from build123d import *

# Parameters (mm, degrees)
SKETCH1_W                       = 16
SKETCH1_H                       = 3.2
BOSS_EXTRUDE1_DEPTH             = 15.8
SKETCH2_R                       = 2.4
BOSS_EXTRUDE2_DEPTH             = 1.6
LPATTERN1_COUNT                 = 2
LPATTERN1_PITCH                 = 8
LPATTERN1_COUNT_DIR2            = 6
LPATTERN1_PITCH_DIR2            = 8
SHELL1_T                        = -1.2
SKETCH3_R                       = 3.25
SKETCH3_R_2                     = 2.4
BOSS_EXTRUDE3_DEPTH             = 1.8
SHELL2_START                    = -14.6
SHELL2_DEPTH                    = 13.4
BOSS_EXTRUDE4_REACH             = 32.137
SKETCH11_R                      = 2.4
SKETCH11_R_2                    = 1.55
BOSS_EXTRUDE4_DIRECTION_2_DEPTH = 1.6
SHELL6_T                        = -1.2


# Read off the part's stored shape, not the designer's step: Shell2
with BuildPart() as part:
    # Sketch1 → Boss-Extrude1 (new body)
    with BuildSketch(Plane.XY):
        with Locations((8, 1.6)):
            Rectangle(SKETCH1_W, SKETCH1_H)
    extrude(amount=-BOSS_EXTRUDE1_DEPTH)

    # Sketch2 → Boss-Extrude2 (add)
    with BuildSketch(Plane(origin=(0, 3.2, 0), x_dir=(1, 0, 0), z_dir=(0, 1, 0))):
        with Locations(Location((3.9, 3.9, 0), (0, 0, 270))):
            Circle(SKETCH2_R)
    boss_extrude2 = extrude(amount=BOSS_EXTRUDE2_DEPTH)

    # LPattern1: Boss-Extrude2 2 × 6, 8 skipped
    with Locations(*[(j * LPATTERN1_PITCH_DIR2, 0, -i * LPATTERN1_PITCH) for i in range(LPATTERN1_COUNT) for j in range(LPATTERN1_COUNT_DIR2) if (i, j) not in ((0, 0), (0, 2), (0, 3), (0, 4), (0, 5), (1, 2), (1, 3), (1, 4), (1, 5))]):
        add(boss_extrude2)

    # Shell1
    shell1_openings = [part.faces().sort_by_distance(p)[0] for p in [
        (8, 0, -7.9),
    ]]
    offset(amount=SHELL1_T, openings=shell1_openings, kind=Kind.INTERSECTION)

    # Sketch3 → Boss-Extrude3 (add)
    with BuildSketch(Plane.XZ.offset(-2)):
        with Locations(Location((7.9, -7.9, 0), (0, 0, 90))):
            Circle(SKETCH3_R)
        with Locations(Location((7.9, -7.9, 0), (0, 0, 270))):
            Circle(SKETCH3_R_2, mode=Mode.SUBTRACT)
    extrude(amount=BOSS_EXTRUDE3_DEPTH)

    # Sketch7 → Loft1 section 0
    with BuildSketch(Plane(origin=(23.8, 0, 0), x_dir=(0, 0, -1), z_dir=(1, 0, 0))):
        with BuildLine():
            Line((15.8, 9.6), (15.8, 8.4))
            Line((15.8, 8.4), (0, 8.4))
            Line((0, 8.4), (0, 9.6))
            Line((0, 9.6), (15.8, 9.6))
        make_face()
    # Sketch5 → Loft1 section 1
    with BuildSketch(Plane(origin=(16, 0, 0), x_dir=(0, 0, -1), z_dir=(1, 0, 0))):
        with BuildLine():
            Line((0, 0), (0, 9.6))
            Line((0, 9.6), (15.8, 9.6))
            Line((15.8, 9.6), (15.8, 0))
            Line((15.8, 0), (0, 0))
        make_face()
    loft1 = loft()

    # Shell2 outline → Shell2 (cut)
    with BuildSketch(Plane.XY.offset(SHELL2_START)):
        Polygon((16, 1.763535985), (16.219573728, 2), (16, 2), align=None)
        Polygon((17.2, 9.6), (17.2, 3.055843678), (22.6, 8.871228293), (22.6, 9.6), align=None)
    extrude(amount=SHELL2_DEPTH, mode=Mode.SUBTRACT)

    # Sketch11 → Boss-Extrude4 (add, up to next)
    with BuildSketch(Plane(origin=(0, 9.6, 0), x_dir=(1, 0, 0), z_dir=(0, 1, 0)), mode=Mode.PRIVATE) as boss_extrude4_sk1:
        with Locations(Location((19.9, 11.9, 0), (0, 0, 180))):
            Circle(SKETCH11_R)
        with Locations((19.9, 11.9)):
            Circle(SKETCH11_R_2, mode=Mode.SUBTRACT)
    boss_extrude4_tool1 = extrude(boss_extrude4_sk1.sketch, amount=-BOSS_EXTRUDE4_REACH, mode=Mode.PRIVATE) - part.part
    # Sketch11 → Boss-Extrude4 (add, up to next)
    with BuildSketch(Plane(origin=(0, 9.6, 0), x_dir=(1, 0, 0), z_dir=(0, 1, 0)), mode=Mode.PRIVATE) as boss_extrude4_sk2:
        with Locations(Location((19.9, 3.9, 0), (0, 0, 180))):
            Circle(SKETCH11_R)
        with Locations((19.9, 3.9)):
            Circle(SKETCH11_R_2, mode=Mode.SUBTRACT)
    boss_extrude4_tool2 = extrude(boss_extrude4_sk2.sketch, amount=-BOSS_EXTRUDE4_REACH, mode=Mode.PRIVATE) - part.part
    boss_extrude4_1 = boss_extrude4_tool1.solids().sort_by_distance((22.232118, 9.6, -11.9))[0]
    add(boss_extrude4_1)
    boss_extrude4_2 = boss_extrude4_tool2.solids().sort_by_distance((22.232118, 9.6, -3.9))[0]
    add(boss_extrude4_2)
    boss_extrude4 = boss_extrude4_1 + boss_extrude4_2  # Boss-Extrude4 as one shape, for the pattern or mirror that repeats it

    # Sketch11 → Boss-Extrude4 direction 2 (add)
    # profile 1 of 2: a face of its own
    with BuildSketch(Plane(origin=(0, 9.6, 0), x_dir=(1, 0, 0), z_dir=(0, 1, 0))):
        with Locations(Location((19.9, 11.9, 0), (0, 0, 180))):
            Circle(SKETCH11_R)
        with Locations((19.9, 11.9)):
            Circle(SKETCH11_R_2, mode=Mode.SUBTRACT)
    # profile 2 of 2: a face of its own
    with BuildSketch(Plane(origin=(0, 9.6, 0), x_dir=(1, 0, 0), z_dir=(0, 1, 0))):
        with Locations(Location((19.9, 3.9, 0), (0, 0, 180))):
            Circle(SKETCH11_R)
        with Locations((19.9, 3.9)):
            Circle(SKETCH11_R_2, mode=Mode.SUBTRACT)
    boss_extrude4_direction_2 = extrude(amount=BOSS_EXTRUDE4_DIRECTION_2_DEPTH)

    # Mirror1: Loft1 across plane
    add(loft1.mirror(Plane(origin=(8, 0, 0), x_dir=(0, 0, 1), z_dir=(1, 0, 0))))


with BuildPart() as body_2:
    # Split1: the piece on the far side of the plane
    add(part.part)
    split(bisect_by=Plane(origin=(0, 0, 0), x_dir=(0, 0, 1), z_dir=(1, 0, 0)), keep=Keep.BOTTOM)

    # Shell6
    shell6_openings = [body_2.faces().sort_by_distance(p)[0] for p in [
        (-3.9, 9.6, -7.9),
    ]]
    offset(amount=SHELL6_T, openings=shell6_openings, kind=Kind.INTERSECTION)


with BuildPart() as part_1:
    add(part.part)

    # Split1
    split(bisect_by=Plane(origin=(0, 0, 0), x_dir=(0, 0, 1), z_dir=(1, 0, 0)), keep=Keep.TOP)


with BuildPart() as body_2_1:
    add(body_2.part)

    # Combine1: union part
    add(part_1.part)

    # Mirror4: Boss-Extrude4, Boss-Extrude4 direction 2 across plane
    add(boss_extrude4.mirror(Plane(origin=(8, 0, 0), x_dir=(0, 0, 1), z_dir=(1, 0, 0))))
    add(boss_extrude4_direction_2.mirror(Plane(origin=(8, 0, 0), x_dir=(0, 0, 1), z_dir=(1, 0, 0))))


solid = body_2_1.part
Verification items for the finished model (mm, model axes). A direction names the side the tool comes from. Give positions to 0.01 mm unless a question says otherwise; leave off trailing zeros. Write each loop counter-clockwise with the first axis right and the second up, starting at its lowest first coordinate (ties: lowest second). Pieces come first, ordered by that corner, then holes. Notation, with made-up numbers: (66, -1) - (119, -1) arc R19 ccw to (119, 25) - close; hole circle Ø5 at (-16.5, -10.75). An arc over 180 degrees is marked (long way). Answer as CSV lines item,"result". Start each with the question number.
1. Depth check by flat-ended pin: pin 1 (1.9 mm diameter, centred on x = 3.9, z = -11.9, fed in from +Y); pin 2 (2 mm diameter, centred on x = 4, y = 4.5, fed in from -Z); pin 3 (1.5 mm diameter, centred on x = -4, z = -7, fed in from -Y). Enter the tip coordinate at first touch or a pass-through.
2. Sectioned sample at B-B (y = 2.75). Record the boundary of the cut face in (x, z), then the cut area to 3 significant figures.
3. Thickness scan on line 1 (Z direction, x = -3.9, y = 8.1); line 2 (X direction, y = 9, z = -6.5); line 3 (Z direction, x = -3.9, y = 9.9). Record the ranges inside material, lowest first.
4. Sectioned sample at A-A (x = 11.9). Record the boundary of the cut face in (y, z), then the cut area to 3 significant figures.
5. Set-up check for faces 1 (the face through (1.557, 3.989, -12.42)), 2 (the face through (8, 1, -1.2)): record each of +Z, -Z, +X, -X, +Y, -Y from which the full face is reachable in a straight line by a thin tool's end or side.
6. Draft check along X on faces 3 (the face through (19.845, 4.141, -8.011)), 4 (the face through (12, 3.6, -4)), 5 (the face through (-1.2, 6, -8)). Enter one of: pulls with the +X half, pulls with the -X half, needs draft (parallel to the pull), parting line crosses it, or undercut.
7. Sectioned sample at D-D (x = -4). Record the boundary of the cut face in (y, z).
Derived:
1,pin 1,"y = 4.8"
1,pin 2,"z = -14.3"
1,pin 3,"y = 3.5"
2,outline,"(-2.55, -15.8) - (18.55, -15.8) - (18.55, 0) - (-2.55, 0) - close; hole circle Ø2.4 at (3.9, -11.9); hole circle Ø2.4 at (3.9, -3.9); hole circle Ø2.4 at (11.9, -11.9); hole circle Ø2.4 at (11.9, -3.9)"
2,area,"315 mm²"
3,line 1,"-15.8 to -14.6, -14.3 to -13.45, -10.35 to -9.5, -6.3 to -5.45, -2.35 to -1.5, -1.2 to 0"
3,line 2,"-7.8 to -6.6, -1.2 to 0, 16 to 17.2, 22.6 to 23.8"
3,line 3,"-14.3 to -13.45, -10.35 to -9.5, -6.3 to -5.45, -2.35 to -1.5"
4,outline,"(0, -15.8) - (3.2, -15.8) - (3.2, -14.3) - (4.8, -14.3) - (4.8, -9.5) - (3.2, -9.5) - (3.2, -6.3) - (4.8, -6.3) - (4.8, -1.5) - (3.2, -1.5) - (3.2, 0) - (0, 0) - (0, -1.2) - (2, -1.2) - (2, -2.7) - (3.6, -2.7) - (3.6, -5.1) - (2, -5.1) - (2, -10.7) - (3.6, -10.7) - (3.6, -13.1) - (2, -13.1) - (2, -14.6) - (0, -14.6) - close"
4,area,"31.4 mm²"
5,face 1,"+Y"
5,face 2,"-Y"
6,face 3,"pulls with the +X half"
6,face 4,"undercut"
6,face 5,"undercut"
7,outline,"(4.31, -15.8) - (9.6, -15.8) - (9.6, -14.6) - (6.07, -14.6) - (6.07, -14.3) - (11.2, -14.3) - (11.2, -13.45) - (6.07, -13.45) - (6.07, -10.35) - (11.2, -10.35) - (11.2, -9.5) - (6.07, -9.5) - (6.07, -6.3) - (11.2, -6.3) - (11.2, -5.45) - (6.07, -5.45) - (6.07, -2.35) - (11.2, -2.35) - (11.2, -1.5) - (6.07, -1.5) - (6.07, -1.2) - (9.6, -1.2) - (9.6, 0) - (4.31, 0) - close"
